```python
from build123d import *

# Parameters (mm, degrees)
SKETCH_1_W          = 32
SKETCH_1_H          = 86
EXTRUDE_1_DEPTH     = 3
SKETCH_2_W          = 12
SKETCH_2_H          = 3
SKETCH_2_W_2        = 3
CUT_EXTRUDE_1_DEPTH = 4
SKETCH_3_W          = 3
SKETCH_3_H          = 10
CUT_EXTRUDE_2_DEPTH = 4
CUT_EXTRUDE_3_DEPTH = 10


with BuildPart() as part:
    # 스케치1 → 보스-돌출1 (new body)
    with BuildSketch(Plane.XY):
        with Locations((16, 43)):
            Rectangle(SKETCH_1_W, SKETCH_1_H)
    extrude(amount=EXTRUDE_1_DEPTH)

    # 스케치2 → 컷-돌출1 (cut, through all)
    with BuildSketch(Plane.XY.offset(3)):
        with Locations((16, 84.5)):
            Rectangle(SKETCH_2_W, SKETCH_2_H)
        with Locations((1.5, 84.5)):
            Rectangle(SKETCH_2_W_2, SKETCH_2_H)
        with Locations((30.5, 84.5)):
            Rectangle(SKETCH_2_W_2, SKETCH_2_H)
        with Locations((16, 1.5)):
            Rectangle(SKETCH_2_W, SKETCH_2_H)
        with Locations((1.5, 1.5)):
            Rectangle(SKETCH_2_W_2, SKETCH_2_H)
        with Locations((30.5, 1.5)):
            Rectangle(SKETCH_2_W_2, SKETCH_2_H)
    extrude(amount=-CUT_EXTRUDE_1_DEPTH, mode=Mode.SUBTRACT)

    # 스케치3 → 컷-돌출2 (cut, through all)
    with BuildSketch(Plane.XY.offset(3)):
        with Locations((27.5, 69)):
            Rectangle(SKETCH_3_W, SKETCH_3_H)
        with Locations((4.5, 69)):
            Rectangle(SKETCH_3_W, SKETCH_3_H)
        with Locations((27.5, 17)):
            Rectangle(SKETCH_3_W, SKETCH_3_H)
        with Locations((4.5, 17)):
            Rectangle(SKETCH_3_W, SKETCH_3_H)
    extrude(amount=-CUT_EXTRUDE_2_DEPTH, mode=Mode.SUBTRACT)

    # 스케치4 → 컷-돌출3 (cut)
    with BuildSketch(Plane.XY.offset(3)):
        Polygon((14.75, 3), (17.25, 3), (17.25, 6.727769783), (18.2, 6.727769783), (18.2, 8.927769783), (17.25, 8.927769783), (17.25, 10), (14.75, 10), (14.75, 8.927769783), (13.8, 8.927769783), (13.8, 6.727769783), (14.75, 6.727769783), align=None)
        Polygon((13.8, 77.072230217), (14.75, 77.072230217), (14.75, 76), (17.25, 76), (17.25, 77.072230217), (18.2, 77.072230217), (18.2, 79.272230217), (17.25, 79.272230217), (17.25, 83), (14.75, 83), (14.75, 79.272230217), (13.8, 79.272230217), align=None)
    extrude(amount=-CUT_EXTRUDE_3_DEPTH, mode=Mode.SUBTRACT)


solid = part.part
```
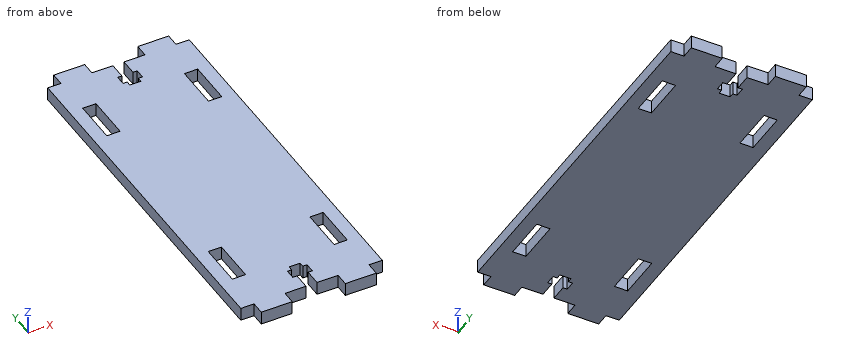
Here's how the part is built. I have some questions about the finished solid (model axes, mm). Round coordinates to 2 decimals unless told otherwise and drop trailing zeros. Order: outer loops, then holes, each group sorted by start corner. A loop starts at its lowest first (then second) coordinate and runs counter-clockwise, first axis right, second up. Notation, with made-up numbers: M 85.25,30 L 135.25,30 A22 cw 135.25,69 Z; hole C 69.5,15.25 d11. An arc over 180 degrees is marked long. Answer in a Markdown table with one row per item.
Item 1: Imagine slicing it at C-C, the plane z = 2.35. State how many separate pieces and enclosed holes the cut face has, and give its area (3 significant figures).
A:
| item | result |
|---|---|
| separate pieces | 1 |
| enclosed holes | 4 |
| area | 2,480 mm2 |
Item 2: Imagine slicing it at D-D, the plane x = 16.5. Write out the boundary of the cut face in (y, z), and give its area (3 significant figures).
A:
| item | result |
|---|---|
| outline | M 10,0 L 76,0 L 76,3 L 10,3 Z |
| area | 198 mm2 |
Item 3: I'm going to push flat-ended pins straight in: pin 1 (0.9 mm diameter, centred on y = 1, z = 2, fed in from -X); pin 2 (1.5 mm diameter, centred on x = 11.5, z = 2, fed in from +Y); pin 3 (0.5 mm diameter, centred on x = 14.5, z = 1.5, fed in from -Y). Where does each tip first touch, or does it pass through?
A:
| item | result |
|---|---|
| pin 1 | stops at x = 3 |
| pin 2 | stops at y = 83 |
| pin 3 | stops at y = 3 |
Item 4: Imagine slicing it at B-B, the plane x = 27. Write out the boundary of the cut face in (y, z), and give its area (3 significant figures).
A:
| item | result |
|---|---|
| outline | M 0,0 L 12,0 L 12,3 L 0,3 Z; M 22,0 L 64,0 L 64,3 L 22,3 Z; M 74,0 L 86,0 L 86,3 L 74,3 Z |
| area | 198 mm2 |
Item 5: If I drill on L1, parallel to Y at x = 5.5, z = 0.9; L2, parallel to X at y = 68, z = 0.8; L3, parallel to Y at x = 14, z = 1.85, over which ranges is the centre line in solid material (lowest first)? Write a range as from..to.
A:
| item | result |
|---|---|
| L1 | y = 0..12, 22..64, 74..86 |
| L2 | x = 0..3, 6..26, 29..32 |
| L3 | y = 3..6.73, 8.93..77.07, 79.27..83 |
Item 6: Imagine slicing it at A-A, the plane y = 70.5. Write out the boundary of the cut face in (x, z).
A:
| item | result |
|---|---|
| outline | M 0,0 L 3,0 L 3,3 L 0,3 Z; M 6,0 L 26,0 L 26,3 L 6,3 Z; M 29,0 L 32,0 L 32,3 L 29,3 Z |
